Part model, mm, in its own coordinate system. Face numbers are marked on the shaded views. Round coordinates to 2 decimals unless told otherwise and drop trailing zeros. Write each loop counter-clockwise with the first axis right and the second up, starting at its lowest first coordinate (ties: lowest second). Pieces come first, ordered by that corner, then holes.
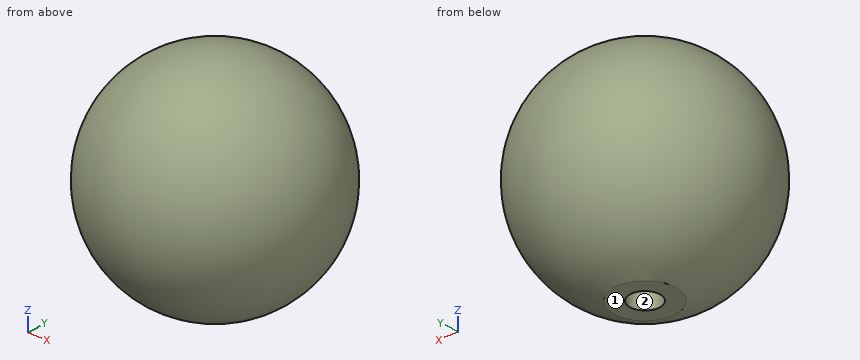
Autodesk Inventor part; units mm, degrees
ref_plane "YZ Plane" through (0, 0, 0) normal (1, 0, 0) x (0, 1, 0)
ref_plane "XZ Plane" through (0, 0, 0) normal (0, 1, 0) x (-1, 0, 0)
sketch "Sketch1" plane through (0, 0, 0) normal (0, 0, 1) x (1, 0, 0)
  circle A0 centre (0, 0) radius 18
  line L0 (-18, 0) -> (18, 0)
  dimension "d0" = 36
  dimension "d1" = 36
revolve "Ball" add sketch "Sketch1" angle 360 about axis through (-18, 0, 0) along (1, 0, 0) picked at (3.4084, 4.9379) contours L0 A0
ref_plane "BottomCuttingPlane" through (0, 0, -17.25) normal (0, 0, 1) x (1, 0, 0)
sketch "CutBottomSketch" plane through (0, 0, -17.25) normal (0, 0, 1) x (1, 0, 0)
  circle A0 centre (0, 0) radius 5.1417
extrude "FlattenBottom" cut sketch "CutBottomSketch" against normal blind 10
sketch "Anchor" plane through (0, 0, -17.25) normal (0, 0, -1) x (-1, 0, 0)
  circle A0 centre (0, 0) radius 5.1417
  circle A1 centre (0, 0) radius 4
  circle A2 centre (0, 0) radius 2.5
  dimension "d6" = 8
  dimension "d7" = 5
extrude "Extrusion2" cut sketch "Anchor" against normal blind 10 contours A2
thread "Thread1"
properties part number "JLF-TP-8YT_ball" material "Acrylic, Clear(1)"
Q1. Drop flat-ended pins along their axis: pin 1 (2.5 mm diameter, centred on x = 1, y = 0, fed in from -Z); pin 2 (6 mm diameter, centred on x = 0, y = 0, fed in from -Z); pin 3 (8 mm diameter, centred on x = 0, y = 0, fed in from +Z). Give the stop position or say it passes through.
Values follow:
pin 1: stops at z = -7.25
pin 2: stops at z = -17.25
pin 3: stops at z = 18
Q2. Wall check: L1, parallel to Y at x = 0, z = -12; L2, parallel to X at y = 0, z = 2.5; L3, parallel to Y at x = -15.5, z = 5.5. Give the ranges that are in metal, low to high.
Values follow:
L1: y = -13.42 to -2.5, 2.5 to 13.42
L2: x = -17.83 to 17.83
L3: y = -7.31 to 7.31
Q3. Cut at C-C on z = 9. Write the cut outline in (x, y), plus the area to 3 significant figures.
Values follow:
outline: circle Ø31.18 at (0, 0)
area: 763 mm2
Q4. Cut at D-D on x = -10.5. Write the cut outline in (y, z), plus the area to 3 significant figures.
Values follow:
outline: circle Ø29.24 at (0, 0)
area: 672 mm2
Q5. Mould opens along X. For the marked faces 1 and 2 say: +X half, -X half, draft (parallel to the pull), parting line (faces both ways), or undercut.
Values follow:
face 1: draft
face 2: undercut
